Work out the finished part from the listing and answer in its coordinate system (mm). Face numbers are marked on the shaded views. A direction names the side the tool comes from. Coordinates: 2 decimals unless noted, no trailing zeros. Order: outer loops, then holes, each group sorted by start corner. A loop starts at its lowest first (then second) coordinate and runs counter-clockwise, first axis right, second up. Notation, with made-up numbers: (21.25, -2) -> (41.25, -2) arc R35 ccw to (41.25, 30) -> close; hole circle Ø11 at (-10.5, -9). An arc over 180 degrees is marked (long way). Use one line per item in the form item = value.
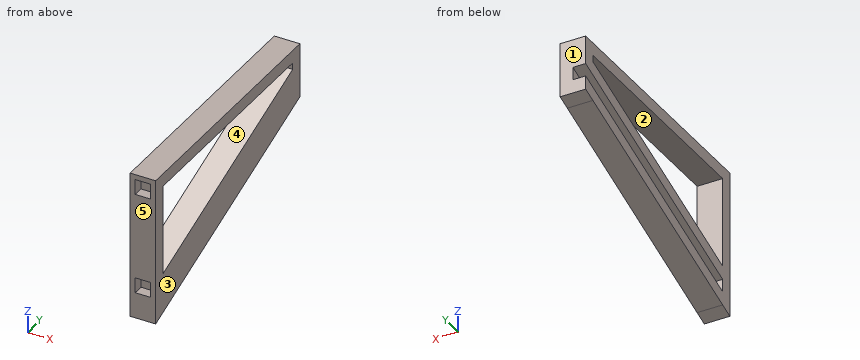
from build123d import *

# Parameters (mm, degrees)
SKETCH1_W           = 100
SKETCH1_H           = 100
BOSS_EXTRUDE1_DEPTH = 10
CUT_EXTRUDE1_DEPTH  = 10
CUT_EXTRUDE2_DEPTH  = 5
SKETCH4_W           = 6
SKETCH4_H           = 6
SKETCH4_W_2         = 3
SKETCH4_H_2         = 3
CUT_EXTRUDE3_DEPTH  = 4
CUT_EXTRUDE4_DEPTH  = 10


with BuildPart() as part:
    # Sketch1 → Boss-Extrude1 (new body)
    with BuildSketch(Plane(origin=(0, 0, 0), x_dir=(0, 0, -1), z_dir=(1, 0, 0))):
        Rectangle(SKETCH1_W, SKETCH1_H)
    extrude(amount=BOSS_EXTRUDE1_DEPTH)

    # Sketch2 → Cut-Extrude1 (cut)
    with BuildSketch(Plane.ZY):
        Polygon((42.398061118, 45), (45, 45), (45, -45), (9.640740034, -45), align=None)
    extrude(amount=-CUT_EXTRUDE1_DEPTH, mode=Mode.SUBTRACT)

    # Sketch2<3> → Cut-Extrude2 (cut)
    with BuildSketch(Plane.ZY):
        Polygon((36.397023427, 50), (33.897023427, 50), (-0.680148829, -45), (4.319851171, -45), (38.897023427, 50), align=None)
    extrude(amount=-CUT_EXTRUDE2_DEPTH, mode=Mode.SUBTRACT)

    # Sketch4 → Cut-Extrude3 (cut)
    with BuildSketch(Plane.XZ.offset(50)):
        with Locations((5, -45)):
            Rectangle(SKETCH4_W, SKETCH4_H)
        with Locations((5, 5.32088886)):
            Rectangle(SKETCH4_W, SKETCH4_H)
        Polygon((8, 42), (8, 45), (5, 45), (5, 48), (2, 48), (2, 42), align=None)
        with Locations((6.5, 46.5)):
            Rectangle(SKETCH4_W_2, SKETCH4_H_2)
        with Locations((6.5, 3.82088886)):
            Rectangle(SKETCH4_W_2, SKETCH4_H_2)
        with Locations((6.5, -46.5)):
            Rectangle(SKETCH4_W_2, SKETCH4_H_2)
    extrude(amount=-CUT_EXTRUDE3_DEPTH, mode=Mode.SUBTRACT)

    # Sketch5 → Cut-Extrude4 (cut)
    with BuildSketch(Plane.ZY):
        Polygon((28.576134564, 50), (-50, 50), (-50, -50), (-7.820888862, -50), (-6.001037691, -45), (26.756283393, 45), align=None)
    extrude(amount=-CUT_EXTRUDE4_DEPTH, mode=Mode.SUBTRACT)


solid = part.part
(1) Which of the six approach directions +Z, -Z, +X, -X, +Y, -Y give full straight-line access (tool end or side, diameter ignored) to the marked faces 4 and 5?
Data:
face_4 = +X, -X
face_5 = +Z, -Z, +X, -X, -Y
(2) The mould has two halves that part along Y. Classify the marked faces 1, 2 and 3: released by +Y, released by -Y, zero draft, split by the parting line, or undercut.
Data:
face_1 = released by +Y
face_2 = undercut
face_3 = zero draft
(3) Section D-D on z = 6.5 is taken. Write down the section's boundary in (x, y), plus the area to 3 significant figures.
Data:
outline = (0, -50) -> (2, -50) -> (2, -46) -> (8, -46) -> (8, -50) -> (10, -50) -> (10, -10.65) -> (0, -10.65) -> (0, -25.27) -> (5, -25.27) -> (5, -39.01) -> (0, -39.01) -> close
area = 301 mm²
(4) Section C-C on y = -18.5 is taken. Write down the section's boundary in (x, z).
Data:
outline = (0, 3.64) -> (10, 3.64) -> (10, 19.29) -> (0, 19.29) -> (0, 13.97) -> (5, 13.97) -> (5, 8.97) -> (0, 8.97) -> close; (0, 45) -> (10, 45) -> (10, 50) -> (0, 50) -> close
(5) Each of these flat-tipped pins is pushed along its axis until it touches: P1, Ø1.8, axis at x = 3.5, z = 4.5, coming from the -Y side; P2, Ø12, axis at y = -14, z = 16, coming from the -X side; P3, Ø1.5, axis at x = 5.5, y = -4.5, coming from the -Z side; P4, Ø1.2, axis at x = 6, y = -47.5, coming from the -Z side. Where does it stop, or does it pass through?
Data:
P1 = -46
P2 = 0
P3 = 8.47
P4 = -7.13
(6) Section A-A on z = 44 is taken. Write down the section's boundary in (x, y), plus the area to 3 significant figures.
Data:
outline = (0, -50) -> (2, -50) -> (2, -46) -> (8, -46) -> (8, -50) -> (10, -50) -> (10, -45) -> (0, -45) -> close; (0, 45) -> (10, 45) -> (10, 50) -> (0, 50) -> close
area = 76.0 mm²
(7) Straight lines are drawn through the part: line 1 along Z through (x, y) = (1.25, 24); line 2 along Z through (x, y) = (3.5, -42); line 3 along Y through (x, z) = (5.75, 43). For each, find the intervals that lie inside material, in ascending order.
Data:
line_1 = 19.11 to 24.43, 29.43 to 34.75, 45 to 50
line_2 = -4.91 to 0.41, 5.41 to 10.73, 45 to 50
line_3 = -46 to -45, 45 to 50
(8) Section B-B on x = 3.5 is taken. Write down the section's boundary in (y, z), plus the area to 3 significant figures.
Data:
outline = (-50, -7.82) -> (50, 28.58) -> (50, 33.9) -> (-45, -0.68) -> (-45, 4.32) -> (50, 38.9) -> (50, 50) -> (-50, 50) -> (-50, 48) -> (-46, 48) -> (-46, 42) -> (-50, 42) -> (-50, 8.32) -> (-46, 8.32) -> (-46, 2.32) -> (-50, 2.32) -> close; hole (-45, 9.64) -> (45, 42.4) -> (45, 45) -> (-45, 45) -> close
area = 1,730 mm²
